```python
from build123d import *

# Parameters (mm, degrees)
SKETCH_W            = 73
SKETCH_H            = 36.5
PAD_DEPTH           = 18.5
SKETCH001_W         = 72
SKETCH001_H         = 14.5
POCKET_DEPTH        = 35.5
SKETCH002_W         = 70
SKETCH002_H         = 2
PAD001_DEPTH        = 3
FILLET_R            = 1
SKETCH003_W         = 2
SKETCH003_H         = 10
PAD002_DEPTH        = 3
FILLET001_R         = 1
SKETCH005_R         = 1.45
PAD003_DEPTH        = 3
CHAMFER_SIZE        = 1
SKETCH006_W         = 20
SKETCH006_H         = 4
POCKET001_DEPTH     = 18.501
LINEARPATTERN_COUNT = 4
LINEARPATTERN_PITCH = 7.666667


with BuildPart() as part:
    # Sketch → Pad (new body)
    with BuildSketch(Plane.XY):
        Rectangle(SKETCH_W, SKETCH_H)
    extrude(amount=PAD_DEPTH)

    # Sketch001 (on Face3 of Pad) → Pocket (cut)
    with BuildSketch(Plane(origin=(0, 18.25, 0), x_dir=(-1, 0, 0), z_dir=(0, 1, 0))):
        with Locations((0.5, 9.25)):
            Rectangle(SKETCH001_W, SKETCH001_H)
    extrude(amount=-POCKET_DEPTH, mode=Mode.SUBTRACT)

    # Sketch002 (on Face9 of Pocket) → Pad001 (join)
    with BuildSketch(Plane.XY.offset(2)):
        with Locations((-1.5, 17.25)):
            Rectangle(SKETCH002_W, SKETCH002_H)
    extrude(amount=PAD001_DEPTH)

    # Fillet
    fillet_edges = [part.edges().sort_by_distance(p)[0] for p in [
        (-1.5, 18.25, 5),
    ]]
    fillet(fillet_edges, radius=FILLET_R)

    # Sketch003 (on Face10 of Fillet) → Pad002 (join)
    with BuildSketch(Plane(origin=(0, 0, 16.5), x_dir=(1, 0, 0), z_dir=(0, 0, -1))):
        with Locations((-35.5, -13.25)):
            Rectangle(SKETCH003_W, SKETCH003_H)
    extrude(amount=PAD002_DEPTH)

    # Fillet001
    fillet001_edges = [part.edges().sort_by_distance(p)[0] for p in [
        (-36.5, 13.25, 13.5),
    ]]
    fillet(fillet001_edges, radius=FILLET001_R)

    # Sketch005 (on Face8 of Fillet001) → Pad003 (join)
    with BuildSketch(Plane.XY.offset(18.5)):
        with Locations((-27.5, 13)):
            Circle(SKETCH005_R)
        with Locations((-27.5, -13)):
            Circle(SKETCH005_R)
        with Locations((27.5, 13)):
            Circle(SKETCH005_R)
        with Locations((27.5, -13)):
            Circle(SKETCH005_R)
    extrude(amount=PAD003_DEPTH)

    # Chamfer
    chamfer_edges = [part.edges().sort_by_distance(p)[0] for p in [
        (26.05, 13, 21.5),
        (-28.95, 13, 21.5),
        (-28.95, -13, 21.5),
        (26.05, -13, 21.5),
    ]]
    chamfer(chamfer_edges, length=CHAMFER_SIZE)

    # Sketch006 (on Face3 of Chamfer) → Pocket001 (cut, through all)
    with BuildSketch(Plane.XY.offset(18.5)):
        with Locations((-13.5, -11.75)):
            Rectangle(SKETCH006_W, SKETCH006_H)
        with Locations((13.5, -11.75)):
            Rectangle(SKETCH006_W, SKETCH006_H)
    pocket001 = extrude(amount=-POCKET001_DEPTH, mode=Mode.SUBTRACT)

    # LinearPattern: Pocket001 ×4
    with Locations(*[(0, i * LINEARPATTERN_PITCH, 0) for i in range(1, LINEARPATTERN_COUNT)]):
        add(pocket001, mode=Mode.SUBTRACT)


solid = part.part
```
Work out the finished part from the listing and answer in its coordinate system (mm). A direction names the side the tool comes from. Round coordinates to 2 decimals unless told otherwise and drop trailing zeros. Order: outer loops, then holes, each group sorted by start corner. A loop starts at its lowest first (then second) coordinate and runs counter-clockwise, first axis right, second up.
Q1. Find the intervals of material crossed by line 1 along X through (y, z) = (5, 18); line 2 along Z through (x, y) = (7, 17); line 3 along Z through (x, y) = (-2, 3), in increasing order.
Solution:
line 1: x = -36.5 to -23.5, -3.5 to 3.5, 23.5 to 36.5
line 2: z = 0 to 5, 16.5 to 18.5
line 3: z = 0 to 2, 16.5 to 18.5
Q2. A tool of negligible diameter and unlimited length cuts with its end or side. For faces 1 (the flat face through (-2, 16.25, 3)), 2 (the cylindrical face through (-26.161, -13.555, 19.486)), 3 (the flat face through (-14, 1.583, 1)), 4 (the flat face through (-1, 0, 0)), from which of +Z, -Z, +X, -X, +Y, -Y can it reach the whole face along a straight path? Write none if from no direction.
Solution:
face 1: -X
face 2: +Z
face 3: +Z, -Z
face 4: -Z, +X, -X, +Y, -Y
Q3. The mould has two halves that part along X. Classify faces 5 (the flat face through (-3.5, 4, 18)), 6 (the flat face through (13, 9.25, 1)), 7 (the flat face through (-2.9, 18.25, 3.8)), 8 (the flat face through (-36.5, 1, 17)): pulls with the +X half, pulls with the -X half, needs draft (parallel to the pull), parting line crosses it, or undercut.
Solution:
face 5: undercut
face 6: undercut
face 7: needs draft
face 8: pulls with the -X half
Q4. A cutting plane is placed at C-C, the plane z = 7. Determine the outline of the cut face in (x, y), then the cut area to 4 significant figures.
Solution:
outline: (-36.5, -18.25) - (36.5, -18.25) - (36.5, 18.25) - (35.5, 18.25) - (35.5, -17.25) - (-36.5, -17.25) - close
area: 108.5 mm2
Q5. A cutting plane is placed at B-B, the plane y = 15.5. Determine the outline of the cut face in (x, z).
Solution:
outline: (-36.5, 0) - (36.5, 0) - (36.5, 18.5) - (-36.5, 18.5) - (-36.5, 14.5) arc R1 ccw to (-35.5, 13.5) - (-34.5, 13.5) - (-34.5, 16.5) - (35.5, 16.5) - (35.5, 2) - (-36.5, 2) - close
Q6. A cutting plane is placed at A-A, the plane y = 2.5. Determine the outline of the cut face in (x, z).
Solution:
outline: (-36.5, 0) - (-23.5, 0) - (-23.5, 2) - (-36.5, 2) - close; (-36.5, 16.5) - (-23.5, 16.5) - (-23.5, 18.5) - (-36.5, 18.5) - close; (-3.5, 0) - (3.5, 0) - (3.5, 2) - (-3.5, 2) - close; (-3.5, 16.5) - (3.5, 16.5) - (3.5, 18.5) - (-3.5, 18.5) - close; (23.5, 0) - (36.5, 0) - (36.5, 18.5) - (23.5, 18.5) - (23.5, 16.5) - (35.5, 16.5) - (35.5, 2) - (23.5, 2) - close
Q7. A cutting plane is placed at D-D, the plane x = -31. Determine the outline of the cut face in (y, z), then the cut area to 3 significant figures.
Solution:
outline: (-18.25, 0) - (18.25, 0) - (18.25, 4) arc R1 ccw to (17.25, 5) - (16.25, 5) - (16.25, 2) - (-17.25, 2) - (-17.25, 16.5) - (18.25, 16.5) - (18.25, 18.5) - (-18.25, 18.5) - close
area: 166 mm2
Q8. Given pin 1 Ø10 at (x, y) = (4, -7) entering from +Z; pin 2 Ø5 at (x, y) = (-26.5, -10) entering from +Z; pin 3 Ø1.5 at (y, z) = (0, 3) entering from -X, each flat-ended and moving along its own axis, determine where each tip first touches the part or whether it passes through.
Solution:
pin 1: stops at z = 18.5
pin 2: stops at z = 21.29
pin 3: stops at x = 35.5
